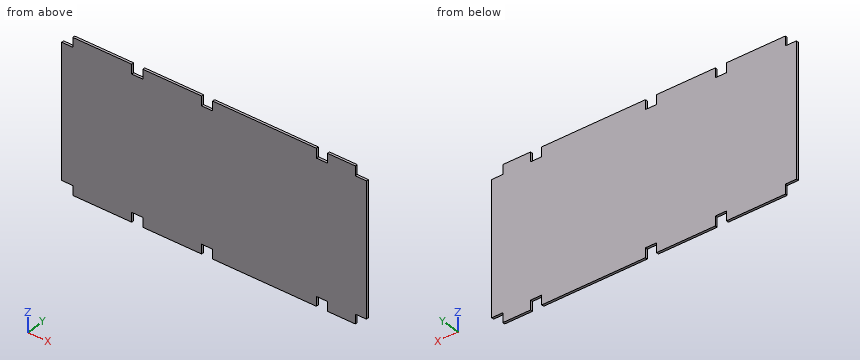
```python
from build123d import *

# Parameters (mm, degrees)
SKETCH1_W           = 2438.4
SKETCH1_H           = 1219.2
BOSS_EXTRUDE1_DEPTH = 9.525
SKETCH2_W           = 88.9
SKETCH2_H           = 76.2
CUT_EXTRUDE1_DEPTH  = 20.05


with BuildPart() as part:
    # Sketch1 → Boss-Extrude1 (new body, symmetric)
    with BuildSketch(Plane(origin=(0, 0, 0), x_dir=(1, 0, 0), z_dir=(0, 1, 0))):
        with Locations((1219.2, 609.6)):
            Rectangle(SKETCH1_W, SKETCH1_H)
    extrude(amount=BOSS_EXTRUDE1_DEPTH, both=True)

    # Sketch2 → Cut-Extrude1 (cut, through all)
    with BuildSketch(Plane(origin=(0, 9.525, 0), x_dir=(1, 0, 0), z_dir=(0, 1, 0))):
        with Locations((44.45, 1181.1)):
            Rectangle(SKETCH2_W, SKETCH2_H)
        with Locations((604.8375, 1181.1)):
            Rectangle(SKETCH2_W, SKETCH2_H)
        with Locations((1163.6375, 1181.1)):
            Rectangle(SKETCH2_W, SKETCH2_H)
        with Locations((2082.8, 1181.1)):
            Rectangle(SKETCH2_W, SKETCH2_H)
        with Locations((2393.95, 1181.1)):
            Rectangle(SKETCH2_W, SKETCH2_H)
        with Locations((1163.6375, 38.1)):
            Rectangle(SKETCH2_W, SKETCH2_H)
        with Locations((604.8375, 38.1)):
            Rectangle(SKETCH2_W, SKETCH2_H)
        with Locations((2393.95, 38.1)):
            Rectangle(SKETCH2_W, SKETCH2_H)
        with Locations((2082.8, 38.1)):
            Rectangle(SKETCH2_W, SKETCH2_H)
        with Locations((44.45, 38.1)):
            Rectangle(SKETCH2_W, SKETCH2_H)
    extrude(amount=-CUT_EXTRUDE1_DEPTH, mode=Mode.SUBTRACT)


solid = part.part
```
For this review, take the finished solid that the model builds, in its own axes (mm). Round coordinates to 2 decimals unless told otherwise and drop trailing zeros. Write each loop counter-clockwise with the first axis right and the second up, starting at its lowest first coordinate (ties: lowest second). Pieces come first, ordered by that corner, then holes.
1) Insertion check: pin 1 Ø9.5 at (x, y) = (600, 3) entering from -Z; pin 2 Ø5.5 at (x, y) = (66.5, -3) entering from +Z; pin 3 Ø9.5 at (y, z) = (2, -1186.5) entering from -X. Each pin has a flat end and moves straight along its axis. Give the tip position at first contact, or say it passes through.
Answer below:
pin 1: stops at z = -1143
pin 2: stops at z = -76.2
pin 3: stops at x = 88.9
2) Take a section at A-A on x = 613.5. Give the boundary of the cut face in (y, z) (3 decimals), then the cut area to 3 significant figures.
Answer below:
outline: (-9.525, -1143) - (9.525, -1143) - (9.525, -76.2) - (-9.525, -76.2) - close
area: 20,300 mm2
3) For line 1 along X through (y, z) = (-4.25, -1160); line 2 along Z through (x, y) = (567.5, -8.5), list the stretches that pass through material, from the lowest coordinate up.
Answer below:
line 1: x = 88.9 to 560.39, 649.29 to 1119.19, 1208.09 to 2038.35, 2127.25 to 2349.5
line 2: z = -1143 to -76.2
